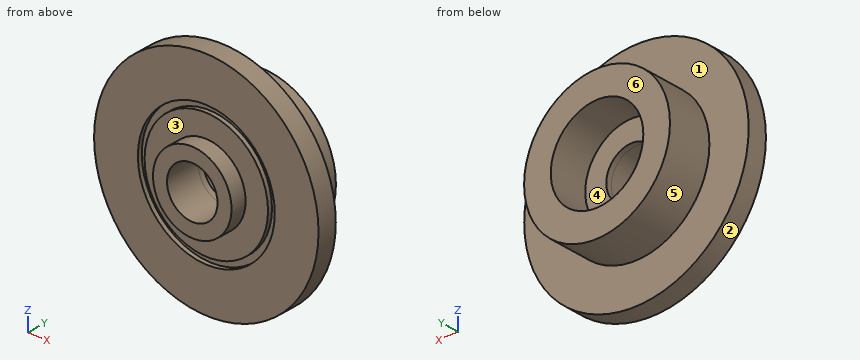
from build123d import *

# Parameters (mm, degrees)
F0_R      = 40
F0_R_2    = 9
F1_DEPTH  = 7
F2_R      = 14
F2_R_2    = 9
F3_DEPTH  = 10
F4_R      = 12.5
F5_DEPTH  = 4.2
F6_R      = 26
F6_R_2    = 9
F7_DEPTH  = 2
F8_R      = 26
F8_R_2    = 16.5
F9_DEPTH  = 14
F11_R     = 14
F12_DEPTH = 4.3
F13_W     = 2.4
F13_H     = 1.6


with BuildPart() as f1:
    # F0 (on Front) → F1 (new body)
    with BuildSketch(Plane.XZ):
        Circle(F0_R)
        Circle(F0_R_2, mode=Mode.SUBTRACT)
    extrude(amount=F1_DEPTH)

    # F2 (on face) → F3 (join)
    with BuildSketch(Plane.XZ.offset(7)):
        Circle(F2_R)
        Circle(F2_R_2, mode=Mode.SUBTRACT)
    extrude(amount=F3_DEPTH)

    # F4 (on face) → F5 (cut)
    with BuildSketch(Plane.XZ.offset(17)):
        Circle(F4_R)
    extrude(amount=-F5_DEPTH, mode=Mode.SUBTRACT)

    # F6 (on face) → F7 (join)
    with BuildSketch(Plane(origin=(0, 0, 0), x_dir=(-1, 0, 0), z_dir=(0, 1, 0))):
        Circle(F6_R)
        Circle(F6_R_2, mode=Mode.SUBTRACT)
    extrude(amount=F7_DEPTH)

    # F8 (on face) → F9 (join)
    with BuildSketch(Plane(origin=(0, 2, 0), x_dir=(-1, 0, 0), z_dir=(0, 1, 0))):
        Circle(F8_R)
        Circle(F8_R_2, mode=Mode.SUBTRACT)
    extrude(amount=F9_DEPTH)

    # F11 (on face) → F12 (cut)
    with BuildSketch(Plane.XZ.offset(17)):
        Circle(F11_R)
    extrude(amount=-F12_DEPTH, mode=Mode.SUBTRACT)

    # F13 (on Top) → F16 (revolve, cut)
    with BuildSketch(Plane.XY):
        with Locations((23.2, -6.2)):
            Rectangle(F13_W, F13_H)
    revolve(axis=Axis((0, -7, 0), (0, -1, 0)), mode=Mode.SUBTRACT)


with BuildPart() as f14_1:
    # F14: copy of F1
    add(f1.part.moved(Location((0, 0, 110.7))))


solid = f1.part
CAD build for the part. Positions are in the model's coordinates, mm. Face numbers are marked on the shaded views. A direction names the side the tool comes from. Round coordinates to 2 decimals unless told otherwise and drop trailing zeros. Loops run counter-clockwise (first coordinate to the right, second up) from the corner with the lowest first, then second, coordinate; pieces in that order, holes last. Notation, with made-up numbers: M -14.75,49.25 L 32.25,49.25 A13 ccw 32.25,69.25 Z; hole C 87,40 d4. An arc over 180 degrees is marked long. One line per question, with ' | ' between items. Start each with the question number.
Item 1: Cut at C-C, the plane y = 6. Write the cut outline in (x, z), plus the area to 3 significant figures.
Item 2: Which spindle directions (+Z, -Z, +X, -X, +Y, -Y) get a long thin tool onto all of the face, cutting with end or side? Do the marked faces 1, 2 and 3. Say none if no direction does.
Item 3: Wall check: line 1 (Z direction, x = 0, y = -6); line 2 (Z direction, x = 0, y = 9.5); line 3 (Y direction, x = 5, z = -37). Give the ranges that are in metal, low to high.
Item 4: Cut at A-A, the plane x = 0. Write the cut outline in (y, z).
Item 5: Two-plate mould, pull along X, no slides. Class the marked faces 4, 5 and 6: pulls with the +X half, pulls with the -X half, needs draft (parallel to the pull), parting line crosses it, or undercut.
Item 6: Cut at D-D, the plane z = 15.5. Write the cut outline in (x, y), plus the area to 3 significant figures.
Item 7: Pin check, flat tips, straight feed: pin 1 Ø2 at (x, z) = (-2, -6) entering from -Y; pin 2 Ø4 at (x, y) = (-8, -8.5) entering from +Z; pin 3 Ø1.5 at (x, y) = (13.5, 3.5) entering from +Z; pin 4 Ø6 at (x, z) = (20, 4.5) entering from -Y. Stop position of each tip, or through.
Item 8: Cut at B-B, the plane z = 0. Write the cut outline in (x, y).
Responses:
1) outline: C 0,0 d52; hole C 0,0 d33 | area: 1,270 mm²
2) face 1: +Y | face 2: +Y, -Y | face 3: -Y
3) line 1: z = -40 to -24.4, -22 to -9, 9 to 22, 24.4 to 40 | line 2: z = -26 to -16.5, 16.5 to 26 | line 3: y = -7 to 0
4) outline: M -12.7,-14 L -7,-14 L -7,-22 L -5.4,-22 L -5.4,-24.4 L -7,-24.4 L -7,-40 L 0,-40 L 0,-26 L 16,-26 L 16,-16.5 L 2,-16.5 L 2,-9 L -12.7,-9 Z; M -12.7,9 L 2,9 L 2,16.5 L 16,16.5 L 16,26 L 0,26 L 0,40 L -7,40 L -7,24.4 L -5.4,24.4 L -5.4,22 L -7,22 L -7,14 L -12.7,14 Z
5) face 4: undercut | face 5: parting line crosses it | face 6: needs draft
6) outline: M -36.87,-7 L -18.84,-7 L -18.84,-5.4 L -15.61,-5.4 L -15.61,-7 L 15.61,-7 L 15.61,-5.4 L 18.84,-5.4 L 18.84,-7 L 36.87,-7 L 36.87,0 L 20.87,0 L 20.87,16 L 5.66,16 L 5.66,2 L -5.66,2 L -5.66,16 L -20.87,16 L -20.87,0 L -36.87,0 Z | area: 1,020 mm²
7) pin 1: passes through | pin 2: stops at z = 39.44 | pin 3: stops at z = 22.66 | pin 4: stops at y = -7
8) outline: M -40,-7 L -24.4,-7 L -24.4,-5.4 L -22,-5.4 L -22,-7 L -14,-7 L -14,-12.7 L -9,-12.7 L -9,2 L -16.5,2 L -16.5,16 L -26,16 L -26,0 L -40,0 Z; M 9,-12.7 L 14,-12.7 L 14,-7 L 22,-7 L 22,-5.4 L 24.4,-5.4 L 24.4,-7 L 40,-7 L 40,0 L 26,0 L 26,16 L 16.5,16 L 16.5,2 L 9,2 Z
